Geometry: final body of the model. Coordinates: model frame, mm. Face numbers are marked on the shaded views. Coordinates: 2 decimals unless noted, no trailing zeros. Order: outer loops, then holes, each group sorted by start corner. A loop starts at its lowest first (then second) coordinate and runs counter-clockwise, first axis right, second up. Notation, with made-up numbers: M 58.25,1.25 L 84.25,1.25 A26 ccw 84.25,24.25 Z; hole C 28,-33 d1. An arc over 180 degrees is marked long. One line per question, with ' | ' between items.
from build123d import *

# Parameters (mm, degrees)
SKETCH1_W           = 20
SKETCH1_H           = 20
BOSS_EXTRUDE1_DEPTH = 20
SKETCH2_R           = 3.1
CUT_EXTRUDE1_DEPTH  = 20
SKETCH3_R           = 5.075
CUT_EXTRUDE2_DEPTH  = 9.3
CHAMFER1_SIZE       = 3
FILLET1_R           = 10


# Some blends are built 0.0001 mm under size
with BuildPart() as part:
    # Sketch1 → Boss-Extrude1 (new body)
    with BuildSketch(Plane(origin=(0, 0, 0), x_dir=(1, 0, 0), z_dir=(0, 1, 0))):
        Rectangle(SKETCH1_W, SKETCH1_H)
    extrude(amount=BOSS_EXTRUDE1_DEPTH)

    # Sketch2 → Cut-Extrude1 (cut)
    with BuildSketch(Plane(origin=(0, 20, 0), x_dir=(1, 0, 0), z_dir=(0, 1, 0))):
        with Locations(Location((0, 0, 0), (0, 0, 270))):
            Circle(SKETCH2_R)
    extrude(amount=-CUT_EXTRUDE1_DEPTH, mode=Mode.SUBTRACT)

    # Sketch3 → Cut-Extrude2 (cut)
    with BuildSketch(Plane.XZ):
        with Locations(Location((0, 0, 0), (0, 0, 270))):
            Circle(SKETCH3_R)
    extrude(amount=-CUT_EXTRUDE2_DEPTH, mode=Mode.SUBTRACT)

    # Chamfer1
    # the kernel refuses this chamfer: 3 mm, written as the material it takes off along each edge
    with BuildSketch(Plane(origin=(0, 9.3, 0), x_dir=(0, 0, 1), z_dir=(-1, 0, 0))) as chamfer1_piece_1_section:
        Polygon((3.1, CHAMFER1_SIZE), (3.1 + CHAMFER1_SIZE, 0), (3.1, 0), align=None)
    chamfer1_piece_1 = revolve(axis=Axis((0, 9.3, 0), (0, 1, 0)), mode=Mode.PRIVATE)
    chamfer1_piece_1 = chamfer1_piece_1 & Plane(origin=(0, 11.321537765, 0), x_dir=(0, 0, -1), z_dir=(0, -1, 0)) * Cylinder(5.075, 25, mode=Mode.PRIVATE)
    add(chamfer1_piece_1, mode=Mode.SUBTRACT)

    # Fillet1
    fillet1_edges = [part.edges().sort_by_distance(p)[0] for p in [
        (10, 10, 10),
        (10, 10, -10),
        (-10, 10, -10),
        (-10, 10, 10),
    ]]
    fillet(fillet1_edges, radius=FILLET1_R - 0.0001)  # a hair under: the kernel refuses the full size


solid = part.part
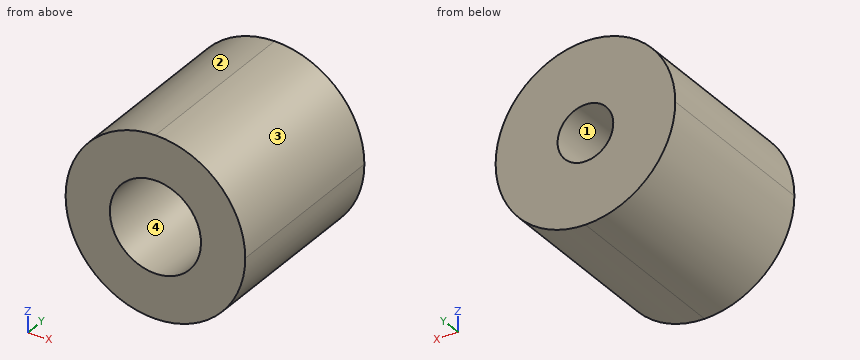
1. Pin query (flat end, axial travel): P1, Ø3, axis at y = 13.5, z = 7, coming from the -X side; P2, Ø3, axis at y = 10, z = 2, coming from the +X side; P3, Ø2, axis at x = -7.5, y = 5.5, coming from the -Z side. Return the tip coordinate at first contact, or that it passes through.
Response values:
P1: stops at x = -8.35 | P2: stops at x = 9.99 | P3: stops at z = -7.6
2. Section C-C, the plane x = 5.75. Output: boundary loops of the cut face in (y, z), and give its area (3 significant figures).
Response values:
outline: M 0,-8.18 L 20,-8.18 L 20,8.18 L 0,8.18 Z | area: 327 mm^2
3. Section D-D, the plane x = 8. Output: boundary loops of the cut face in (y, z).
Response values:
outline: M 0,-6 L 20,-6 L 20,6 L 0,6 Z
4. Draft query along X for the marked faces 1, 2, 3 and 4. Return one class per face: pulls with the +X half, pulls with the -X half, needs draft (parallel to the pull), parting line crosses it, or undercut.
Response values:
face 1: undercut | face 2: pulls with the -X half | face 3: pulls with the +X half | face 4: undercut
5. Material intervals for line 1 (X direction, y = 7, z = 0) (3 decimals); line 2 (X direction, y = 15.5, z = 0), sorted ascending. Write a range as [from, to].
Response values:
line 1: x = [-10, -5.075], [5.075, 10] | line 2: x = [-10, -3.1], [3.1, 10]
